Read the model definition and answer for the solid it produces. Units are mm, in the model's axes. Round coordinates to 2 decimals unless told otherwise and drop trailing zeros. Write each loop counter-clockwise with the first axis right and the second up, starting at its lowest first coordinate (ties: lowest second). Pieces come first, ordered by that corner, then holes. Notation, with made-up numbers: (34.25, 65.5) -> (80.25, 65.5) arc R19 ccw to (80.25, 81.5) -> close; hole circle Ø11 at (-1.5, 32.5). An arc over 180 degrees is marked (long way). Return JSON: item names as keys, results as strings. Group by question number.
(1) The mould has two halves that part along X. Classify faces 1 (the cylindrical face through (-7.493, -0.28, 0.33)), 2 (the flat face through (-60, 0, 5)), 3 (the flat face through (15, 0, 5)): released by +X, released by -X, zero draft, split by the parting line, or undercut.
(2) Straight lines are drawn through the part: line 1 (Z direction, x = 0, y = 1); line 2 (X direction, y = 17.5, z = 4.5); line 3 (Z direction, x = -1, y = -10.5). For each, find the intervals that lie inside material, in ascending order.
(3) A cutting plane is placed at C-C on y = 11.5. Give the vertices of the cut face in (x, z), then the cut area to 3 significant figures.
(4) A cutting plane is placed at B-B on x = 0. Give the vertices of the cut face in (y, z), then the cut area to 3 significant figures.
(5) A cutting plane is placed at A-A on z = 0. Give the vertices of the cut face in (x, y).
```python
from build123d import *

# Parameters (mm, degrees)
F0_W     = 75
F0_H     = 50
F1_DEPTH = 20
F2_R     = 7.5
F3_DEPTH = 40


with BuildPart() as f1:
    # F0 (on Front) → F1 (new body, symmetric)
    with BuildSketch(Plane.XZ):
        with Locations((-22.5, 5)):
            Rectangle(F0_W, F0_H)
    extrude(amount=F1_DEPTH, both=True)

    # F2 (on face) → F3 (cut, through all)
    with BuildSketch(Plane.XZ.offset(20)):
        Circle(F2_R)
    extrude(amount=-F3_DEPTH, mode=Mode.SUBTRACT)


solid = f1.part
```
Checks:
{
 "1": {"face 1": "undercut", "face 2": "released by -X", "face 3": "released by +X"},
 "2": {"line 1": "z = -20 to -7.5, 7.5 to 30", "line 2": "x = -60 to -6, 6 to 15", "line 3": "z = -20 to -7.43, 7.43 to 30"},
 "3": {"outline": "(-60, -20) -> (15, -20) -> (15, 30) -> (-60, 30) -> close; hole circle Ø15 at (0, 0)", "area": "3,570 mm^2"},
 "4": {"outline": "(-20, -20) -> (20, -20) -> (20, -7.5) -> (-20, -7.5) -> close; (-20, 7.5) -> (20, 7.5) -> (20, 30) -> (-20, 30) -> close", "area": "1,400 mm^2"},
 "5": {"outline": "(-60, -20) -> (-7.5, -20) -> (-7.5, 20) -> (-60, 20) -> close; (7.5, -20) -> (15, -20) -> (15, 20) -> (7.5, 20) -> close"}
}
